Autodesk Inventor part; units mm, degrees
ref_plane "YZ Plane" through (0, 0, 0) normal (1, 0, 0) x (0, 1, 0)
ref_plane "XZ Plane" through (0, 0, 0) normal (0, 1, 0) x (-1, 0, 0)
ref_plane "XY Plane" through (0, 0, 0) normal (0, 0, 1) x (1, 0, 0)
sketch "Sketch1" plane through (0, 0, 0) normal (1, 0, 0) x (0, 1, 0)
  circle A0 centre (0, 0) radius 2.5
  dimension "d0" = 5
extrude "Extrusion1" add sketch "Sketch1" along normal blind 71
sketch "Sketch2" plane through (71, 0, 0) normal (1, 0, 0) x (0, 0, -1)
  circle A0 centre (0, 0) radius 2.5
  arc A1 (0, -2.5) -> (0, 2.5) centre (0, 0) ccw
  line L0 (0, -2.5) -> (0, 2.5)
extrude "Extrusion2" cut sketch "Sketch2" against normal blind 7 contours A0 L0 picked at (0.5196, 0.6515)
sketch "Sketch3" plane through (0, 0, 0) normal (-1, 0, 0) x (0, 0, 1)
  arc A0 (0, 2.5) -> (0, -2.5) centre (0, 0) ccw
  circle A1 centre (0, 0) radius 2.5
  arc A2 (0, -2.5) -> (0, 2.5) centre (0, 0) ccw
  arc A3 (0, -2.5) -> (0, 2.5) centre (0, 0) ccw
  line L0 (0, -2.5) -> (0, 2.5)
extrude "Extrusion3" cut sketch "Sketch3" against normal blind 7 contours A1 L0
properties part number "Aluminum_Rod_70mm"
Source: CAD feature listing. Evaluate the final solid. Frame: model axes, mm. A direction names the side the tool comes from. Coordinates: 2 decimals unless noted, no trailing zeros. Order: outer loops, then holes, each group sorted by start corner. A loop starts at its lowest first (then second) coordinate and runs counter-clockwise, first axis right, second up. Notation, with made-up numbers: M 6,76 L 60,76 A20 ccw 60,98 Z; hole C -3,46 d7. An arc over 180 degrees is marked long. Write each question's results on one line, items separated by ' | '. Start each with the question number.
Item 1: Cut plane A-A (y = 0). Return loops of the section in (x, z), and give its area (3 significant figures).
Item 2: First-contact query: pin 1 Ø2.5 at (x, y) = (67, 0) entering from -Z; pin 2 Ø3 at (y, z) = (-2, -2) entering from +X; pin 3 Ø1.5 at (x, y) = (23.5, 1.5) entering from +Z. Flat tips, straight axial feed; report the tip coordinate or a pass-through.
Item 3: Line query: probe 1 along Y at (x, z) = (29, -0.25); probe 2 along X at (y, z) = (-1.2, 1.6); probe 3 along X at (y, z) = (-0.2, -0.3). Output: solid intervals per line, ascending.
Item 4: Set-up query: faces 3 (the face through (0, 0, -1)), 4 (the face through (68, 0, 0)), 5 (the face through (7, 0, 1)). Return all of +Z, -Z, +X, -X, +Y, -Y with unobstructed straight access to the full face (end or side cutting, diameter ignored); none if empty.
Item 5: Cut plane B-B (x = 24.5). Return loops of the section in (y, z).
Item 6: Draft query along Y for faces 1 (the face through (35, -0.54, 2.44)), 2 (the face through (71, 0, 1)). Return one class per face: pulls with the +Y half, pulls with the -Y half, needs draft (parallel to the pull), parting line crosses it, or undercut.
Item 7: Cut plane C-C (z = -1). Return loops of the section in (x, y).
Checked values:
1) outline: M 0,-2.5 L 64,-2.5 L 64,0 L 71,0 L 71,2.5 L 7,2.5 L 7,0 L 0,0 Z | area: 320 mm2
2) pin 1: stops at z = 0 | pin 2: stops at x = 64 | pin 3: stops at z = 2.38
3) probe 1: y = -2.49 to 2.49 | probe 2: x = 7 to 71 | probe 3: x = 0 to 64
4) face 3: +Z, -Z, -X, +Y, -Y | face 4: -Z, +X, +Y, -Y | face 5: +Z, -X, +Y, -Y
5) outline: C 0,0 d5
6) face 1: parting line crosses it | face 2: needs draft
7) outline: M 0,-2.29 L 64,-2.29 L 64,2.29 L 0,2.29 Z
